Autodesk Inventor part; units mm, degrees
ref_plane "YZ Plane" through (0, 0, 0) normal (1, 0, 0) x (0, 1, 0)
ref_plane "XZ Plane" through (0, 0, 0) normal (0, 1, 0) x (-1, 0, 0)
ref_plane "XY Plane" through (0, 0, 0) normal (0, 0, 1) x (1, 0, 0)
sketch "Sketch1" plane through (0, 0, 0) normal (0, 1, 0) x (-1, 0, 0)
  line L0 (0, 0) -> (57.15, 0)
  line L1 (57.15, 0) -> (57.15, -19.05)
  line L2 (57.15, -19.05) -> (0, -19.05)
  line L3 (0, -19.05) -> (0, 0)
  circle A0 centre (6.35, -9.525) radius 3.175
  circle A1 centre (50.8, -9.525) radius 3.175
  circle A2 centre (31.75, -9.525) radius 4.7625
  dimension "d0" = 57.15
  dimension "d1" = 19.05
  dimension "d2" = 6.35
  dimension "d3" = 6.35
  dimension "d4" = 9.525
  dimension "d5" = 6.35
  dimension "d6" = 6.35
  dimension "d7" = 9.525
  dimension "d12" = 9.525
  dimension "d13" = 31.75
  dimension "d14" = 9.525
extrude "Extrusion1" add sketch "Sketch1" along normal blind 3.175 contours L0 L1 L2 L3 | A2
extrude "Extrusion2" cut sketch "Sketch1" along normal blind 3.175 contours A2
properties part number "15102898-16-P-0224"
For this review, take the finished solid that the model builds, in its own axes (mm). Give positions to 0.01 mm unless a question says otherwise; leave off trailing zeros. Write each loop counter-clockwise with the first axis right and the second up, starting at its lowest first coordinate (ties: lowest second). Pieces come first, ordered by that corner, then holes. Notation, with made-up numbers: (-4.75, 71.5) -> (17.25, 71.5) arc R19 cw to (17.25, 97.5) -> close; hole circle Ø3 at (53, -37). An arc over 180 degrees is marked (long way). Use CSV: the item, a comma, the result in double quotes.
Q1. Take a section at C-C, the plane y = 1.3. State how many separate pieces and enclosed holes the cut face has, then the cut area to 3 significant figures.
Conclusion:
separate pieces,"1"
enclosed holes,"3"
area,"954 mm2"
Q2. To check wall thickness, follow probe 1 along Z at (x, y) = (-31.75, 1.45); probe 2 along X at (y, z) = (1, -9.5); probe 3 along Z at (x, y) = (-6.35, 2.5). State the ranges of each line that lie inside material, in increasing order. Write a range as [from, to].
Conclusion:
probe 1,"[-19.05, -14.29], [-4.76, 0]"
probe 2,"[-57.15, -53.97], [-47.63, -36.51], [-26.99, -9.52], [-3.18, 0]"
probe 3,"[-19.05, -12.7], [-6.35, 0]"
Q3. Mouldability with a two-part tool opening along Z and no side actions: class faces 1 (the face through (-28, 2, 0)), 2 (the face through (-57.15, 2, -9)), 3 (the face through (-4.01, 1.57, -11.67)) as pulls with the +Z half, pulls with the -Z half, needs draft (parallel to the pull), parting line crosses it, or undercut.
Conclusion:
face 1,"pulls with the +Z half"
face 2,"needs draft"
face 3,"undercut"
Q4. Take a section at D-D, the plane x = -50.8. Write out the cut boundary in (y, z) (3 decimals), then the cut area to 3 significant figures.
Conclusion:
outline,"(0, -19.05) -> (3.175, -19.05) -> (3.175, -12.7) -> (0, -12.7) -> close; (0, -6.35) -> (3.175, -6.35) -> (3.175, 0) -> (0, 0) -> close"
area,"40.3 mm2"
Q5. Take a section at B-B, the plane z = -11.25. Write out the cut boundary in (x, y) (3 decimals), then the cut area to 3 significant figures.
Conclusion:
outline,"(-57.15, 0) -> (-53.466, 0) -> (-53.466, 3.175) -> (-57.15, 3.175) -> close; (-48.134, 0) -> (-36.189, 0) -> (-36.189, 3.175) -> (-48.134, 3.175) -> close; (-27.311, 0) -> (-9.016, 0) -> (-9.016, 3.175) -> (-27.311, 3.175) -> close; (-3.684, 0) -> (0, 0) -> (0, 3.175) -> (-3.684, 3.175) -> close"
area,"119 mm2"
